Source: CAD feature listing. Evaluate the final solid. Frame: model axes, mm. Face numbers are marked on the shaded views. A direction names the side the tool comes from. Round coordinates to 2 decimals unless told otherwise and drop trailing zeros. Order: outer loops, then holes, each group sorted by start corner. A loop starts at its lowest first (then second) coordinate and runs counter-clockwise, first axis right, second up. Notation, with made-up numbers: (57, -30.75) -> (83, -30.75) arc R22 cw to (83, -10.75) -> close; hole circle Ø6 at (48, 52). An arc over 180 degrees is marked (long way). Use a Markdown table: item, result. Add a question column.
```python
from build123d import *

# Parameters (mm, degrees)
ESBO_O1_W                = 24
ESBO_O1_H                = 28
ESBO_O1_R                = 1.5
RESSALTO_EXTRUS_O1_DEPTH = 16
ESBO_O2_W                = 6.1
ESBO_O2_H                = 11.95
CORTE_EXTRUS_O1_DEPTH    = 41.199502484
CORTE_EXTRUS_O3_DEPTH    = 41.199502484
ESBO_O4_R                = 1.5
CORTE_EXTRUS_O4_DEPTH    = 7
CORTE_EXTRUS_O5_DEPTH    = 9
ESBO_O6_R                = 1.5
RESSALTO_EXTRUS_O2_DEPTH = 2


with BuildPart() as part:
    # Esboço1 → Ressalto-extrusão1 (new body)
    with BuildSketch(Plane.XY):
        with Locations((12, 14)):
            Rectangle(ESBO_O1_W, ESBO_O1_H)
        with Locations((12, 19.85)):
            Circle(ESBO_O1_R, mode=Mode.SUBTRACT)
        with Locations((12, 8.15)):
            Circle(ESBO_O1_R, mode=Mode.SUBTRACT)
    extrude(amount=RESSALTO_EXTRUS_O1_DEPTH)

    # Esboço2 → Corte-extrusão1 (cut, through all)
    with BuildSketch(Plane(origin=(0, 0, 0), x_dir=(1, 0, 0), z_dir=(0, 1, 0))):
        with Locations((12, -10.025)):
            Rectangle(ESBO_O2_W, ESBO_O2_H)
        Polygon((0, -13.5), (6.15, -9.1), (6.15, -6.9), (0, -2.5), align=None)
        Polygon((17.85, -6.9), (24, -2.5), (24, -13.5), (17.85, -9.1), align=None)
    extrude(amount=CORTE_EXTRUS_O1_DEPTH, mode=Mode.SUBTRACT)

    # Esboço3 → Corte-extrusão3 (cut, through all)
    with BuildSketch(Plane(origin=(0, 0, 0), x_dir=(0, 0, -1), z_dir=(1, 0, 0))):
        Polygon((-13.5, 28), (-9.1, 23.2), (-6.9, 23.2), (-2.5, 28), align=None)
    extrude(amount=CORTE_EXTRUS_O3_DEPTH, mode=Mode.SUBTRACT)

    # Esboço4 → Corte-extrusão4 (cut)
    with BuildSketch(Plane.XY.offset(16)):
        with Locations((4, 12.1)):
            Circle(ESBO_O4_R)
        with Locations((20, 12.1)):
            Circle(ESBO_O4_R)
    extrude(amount=-CORTE_EXTRUS_O4_DEPTH, mode=Mode.SUBTRACT)

    # Esboço5 → Corte-extrusão5 (cut)
    with BuildSketch(Plane.XY.offset(16)):
        Polygon((4, 8.95), (6.727980022, 10.525), (6.727980022, 13.675), (4, 15.25), (1.272019978, 13.675), (1.272019978, 10.525), align=None)
        Polygon((20, 8.95), (22.727980022, 10.525), (22.727980022, 13.675), (20, 15.25), (17.272019978, 13.675), (17.272019978, 10.525), align=None)
    extrude(amount=-CORTE_EXTRUS_O5_DEPTH, mode=Mode.SUBTRACT)

    # Esboço6 → Ressalto-extrusão2 (add)
    # profile 1 of 2: a face of its own
    with BuildSketch(Plane.XY.offset(16)):
        Polygon((6.727980022, 10.525), (4, 8.95), (1.272019978, 10.525), (1.272019978, 13.675), (4, 15.25), (6.727980022, 13.675), align=None)
        with Locations((4, 12.1)):
            Circle(ESBO_O6_R, mode=Mode.SUBTRACT)
    # profile 2 of 2: a face of its own
    with BuildSketch(Plane.XY.offset(16)):
        Polygon((17.272019978, 13.675), (17.272019978, 10.525), (20, 8.95), (22.727980022, 10.525), (22.727980022, 13.675), (20, 15.25), align=None)
        with Locations((20, 12.1)):
            Circle(ESBO_O6_R, mode=Mode.SUBTRACT)
    extrude(amount=-RESSALTO_EXTRUS_O2_DEPTH)


solid = part.part
```
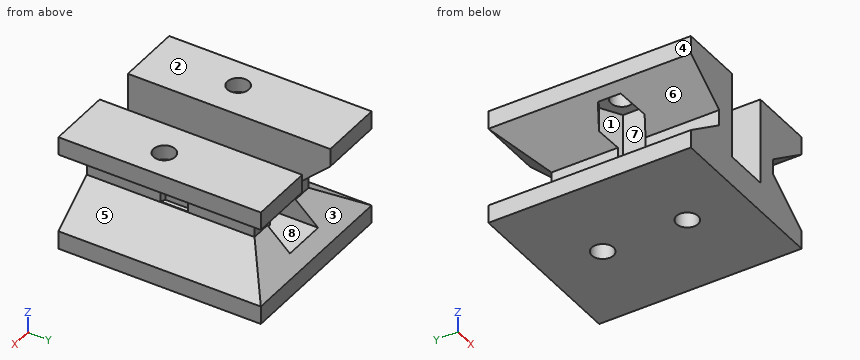
1) First-contact query: pin 1 Ø1.8 at (y, z) = (11, 8) entering from +X; pin 2 Ø2.5 at (x, z) = (7, 8.5) entering from +Y; pin 3 Ø1.6 at (y, z) = (12.5, 9) entering from -X; pin 4 Ø4 at (y, z) = (19, 2) entering from -X. Flat tips, straight axial feed; report the tip coordinate or a pass-through.
2) Draft query along Z for the marked faces 1, 2, 3 and 4. Return one class per face: pulls with the +Z half, pulls with the -Z half, needs draft (parallel to the pull), parting line crosses it, or undercut.
3) Section A-A on x = 12. Output: boundary loops of the cut face in (y, z), then the cut area to 3 significant figures.
4) Reachability of the marked faces 5, 6, 7 and 8 from +Z, -Z, +X, -X, +Y, -Y: full face, straight path, thin tool, end or side. Return the list, or none.
5) Section D-D on z = 1. Output: boundary loops of the cut face in (x, y).
6) Section C-C on y = 12.1. Count the separate pieces of the cut face and the enclosed holes in it, then the cut area to 3 significant figures.
7) Section B-B on y = 8.15. Output: boundary loops of the cut face in (x, z).
8) Line query: probe 1 along Y at (x, z) = (12, 2.45); probe 2 along X at (y, z) = (8.15, 2.1); probe 3 along X at (y, z) = (2, 9). Output: solid intervals per line, ascending. Write a range as from..to.
Conclusion:
| question | item | result |
|---|---|---|
| 1 | pin 1 | stops at x = 17.85 |
| 1 | pin 2 | stops at y = 23.91 |
| 1 | pin 3 | stops at x = 6.73 |
| 1 | pin 4 | stops at x = 0 |
| 2 | face 1 | undercut |
| 2 | face 2 | pulls with the +Z half |
| 2 | face 3 | undercut |
| 2 | face 4 | needs draft |
| 3 | outline | (0, 0) -> (6.65, 0) -> (6.65, 4.05) -> (0, 4.05) -> close; (9.65, 0) -> (18.35, 0) -> (18.35, 4.05) -> (9.65, 4.05) -> close; (21.35, 0) -> (28, 0) -> (28, 2.5) -> (26.31, 4.05) -> (21.35, 4.05) -> close |
| 3 | area | 87.8 mm^2 |
| 4 | face 5 | +X, +Y, -Y |
| 4 | face 6 | -X, +Y, -Y |
| 4 | face 7 | none |
| 4 | face 8 | +Z, +Y, -Y |
| 5 | outline | (0, 0) -> (24, 0) -> (24, 28) -> (0, 28) -> close; hole circle Ø3 at (12, 8.15); hole circle Ø3 at (12, 19.85) |
| 6 | separate pieces | 3 |
| 6 | enclosed holes | 0 |
| 6 | area | 179 mm^2 |
| 7 | outline | (0, 0) -> (10.5, 0) -> (10.5, 4.05) -> (8.95, 4.05) -> (8.95, 16) -> (0, 16) -> (0, 13.5) -> (6.15, 9.1) -> (6.15, 6.9) -> (0, 2.5) -> close; (13.5, 0) -> (24, 0) -> (24, 2.5) -> (17.85, 6.9) -> (17.85, 9.1) -> (24, 13.5) -> (24, 16) -> (15.05, 16) -> (15.05, 4.05) -> (13.5, 4.05) -> close |
| 8 | probe 1 | y = 0..6.65, 9.65..18.35, 21.35..28 |
| 8 | probe 2 | x = 0..10.5, 13.5..24 |
| 8 | probe 3 | x = 6.15..8.95, 15.05..17.85 |
